Can you work these out from the model? Positions are in its coordinate system, mm. A direction names the side the tool comes from. Coordinates: 2 decimals unless noted, no trailing zeros. Loops run counter-clockwise (first coordinate to the right, second up) from the corner with the lowest first, then second, coordinate; pieces in that order, holes last.
```python
from build123d import *

# Parameters (mm, degrees)
SKETCH_1_W          = 60
SKETCH_1_H          = 65
EXTRUDE_1_DEPTH     = 6
SKETCH_2_W          = 60
SKETCH_2_H          = 6
EXTRUDE_2_DEPTH     = 19
CUT_EXTRUDE_2_REACH = 93.924
SKETCH_4_R          = 3
CUT_EXTRUDE_3_REACH = 93.924
SKETCH_3_R          = 27
SKETCH_3_R_2        = 2


with BuildPart() as part:
    # 草圖1 → 填料-伸長1 (new body)
    with BuildSketch(Plane.XY):
        with Locations((30, 32.5)):
            Rectangle(SKETCH_1_W, SKETCH_1_H)
    extrude(amount=EXTRUDE_1_DEPTH)

    # 草圖2 → 填料-伸長2 (add)
    with BuildSketch(Plane.XY.offset(6)):
        with Locations((30, 3)):
            Rectangle(SKETCH_2_W, SKETCH_2_H)
    extrude(amount=EXTRUDE_2_DEPTH)

    # 草圖4 → 除料-伸長2 (cut, up to next)
    with BuildSketch(Plane(origin=(0, 0, 0), x_dir=(-1, 0, 0), z_dir=(0, -1, 0)), mode=Mode.PRIVATE) as cut_extrude_2_sk1:
        with Locations(Location((-13, -12.5, 0), (0, 0, 90))):
            Circle(SKETCH_4_R)
    cut_extrude_2_tool1 = extrude(cut_extrude_2_sk1.sketch, amount=-CUT_EXTRUDE_2_REACH, mode=Mode.PRIVATE) & part.part
    # 草圖4 → 除料-伸長2 (cut, up to next)
    with BuildSketch(Plane(origin=(0, 0, 0), x_dir=(-1, 0, 0), z_dir=(0, -1, 0)), mode=Mode.PRIVATE) as cut_extrude_2_sk2:
        with Locations(Location((-47, -12.5, 0), (0, 0, 90))):
            Circle(SKETCH_4_R)
    cut_extrude_2_tool2 = extrude(cut_extrude_2_sk2.sketch, amount=-CUT_EXTRUDE_2_REACH, mode=Mode.PRIVATE) & part.part
    add(cut_extrude_2_tool1.solids().sort_by_distance((13, 0, 12.5))[0], mode=Mode.SUBTRACT)
    add(cut_extrude_2_tool2.solids().sort_by_distance((47, 0, 12.5))[0], mode=Mode.SUBTRACT)

    # 草圖3 → 除料-伸長3 (cut, up to next)
    with BuildSketch(Plane(origin=(0, 0, 0), x_dir=(-1, 0, 0), z_dir=(0, 0, -1)), mode=Mode.PRIVATE) as cut_extrude_3_sk1:
        with Locations((-30, 35)):
            Circle(SKETCH_3_R)
    cut_extrude_3_tool1 = extrude(cut_extrude_3_sk1.sketch, amount=-CUT_EXTRUDE_3_REACH, mode=Mode.PRIVATE) & part.part
    # 草圖3 → 除料-伸長3 (cut, up to next)
    with BuildSketch(Plane(origin=(0, 0, 0), x_dir=(-1, 0, 0), z_dir=(0, 0, -1)), mode=Mode.PRIVATE) as cut_extrude_3_sk2:
        with Locations((-54.748737342, 59.748737342)):
            Circle(SKETCH_3_R_2)
    cut_extrude_3_tool2 = extrude(cut_extrude_3_sk2.sketch, amount=-CUT_EXTRUDE_3_REACH, mode=Mode.PRIVATE) & part.part
    # 草圖3 → 除料-伸長3 (cut, up to next)
    with BuildSketch(Plane(origin=(0, 0, 0), x_dir=(-1, 0, 0), z_dir=(0, 0, -1)), mode=Mode.PRIVATE) as cut_extrude_3_sk3:
        with Locations((-5.251262658, 59.748737342)):
            Circle(SKETCH_3_R_2)
    cut_extrude_3_tool3 = extrude(cut_extrude_3_sk3.sketch, amount=-CUT_EXTRUDE_3_REACH, mode=Mode.PRIVATE) & part.part
    # 草圖3 → 除料-伸長3 (cut, up to next)
    with BuildSketch(Plane(origin=(0, 0, 0), x_dir=(-1, 0, 0), z_dir=(0, 0, -1)), mode=Mode.PRIVATE) as cut_extrude_3_sk4:
        with Locations((-54.748737342, 10.251262658)):
            Circle(SKETCH_3_R_2)
    cut_extrude_3_tool4 = extrude(cut_extrude_3_sk4.sketch, amount=-CUT_EXTRUDE_3_REACH, mode=Mode.PRIVATE) & part.part
    # 草圖3 → 除料-伸長3 (cut, up to next)
    with BuildSketch(Plane(origin=(0, 0, 0), x_dir=(-1, 0, 0), z_dir=(0, 0, -1)), mode=Mode.PRIVATE) as cut_extrude_3_sk5:
        with Locations((-5.251262658, 10.251262658)):
            Circle(SKETCH_3_R_2)
    cut_extrude_3_tool5 = extrude(cut_extrude_3_sk5.sketch, amount=-CUT_EXTRUDE_3_REACH, mode=Mode.PRIVATE) & part.part
    add(cut_extrude_3_tool1.solids().sort_by_distance((30, 35, 0))[0], mode=Mode.SUBTRACT)
    add(cut_extrude_3_tool2.solids().sort_by_distance((54.748737, 59.748737, 0))[0], mode=Mode.SUBTRACT)
    add(cut_extrude_3_tool3.solids().sort_by_distance((5.251263, 59.748737, 0))[0], mode=Mode.SUBTRACT)
    add(cut_extrude_3_tool4.solids().sort_by_distance((54.748737, 10.251263, 0))[0], mode=Mode.SUBTRACT)
    add(cut_extrude_3_tool5.solids().sort_by_distance((5.251263, 10.251263, 0))[0], mode=Mode.SUBTRACT)


solid = part.part
```
(1) I want a section at D-D on z = 2.25. Write out the boundary of the cut face in (x, y), then the cut area to 3 significant figures.
Check values:
outline: (0, 0) - (60, 0) - (60, 65) - (0, 65) - close; hole circle Ø54 at (30, 35); hole circle Ø4 at (5.25, 10.25); hole circle Ø4 at (5.25, 59.75); hole circle Ø4 at (54.75, 10.25); hole circle Ø4 at (54.75, 59.75)
area: 1,560 mm2
(2) I'm going to push flat-ended pins straight in: pin 1 (6 mm diameter, centred on x = 40.5, z = 16.5, fed in from +Y); pin 2 (5 mm diameter, centred on x = 13, z = 12.5, fed in from -Y). Where does each tip first touch, or does it pass through?
Check values:
pin 1: stops at y = 6
pin 2: passes through
(3) If I drill on probe 1 along X at (y, z) = (1.35, 12.5); probe 2 along X at (y, z) = (10, 5); probe 3 along Y at (x, z) = (15, 18), over which ranges is the centre line in solid material (lowest first)?
Check values:
probe 1: x = 0 to 10, 16 to 44, 50 to 60
probe 2: x = 0 to 3.27, 7.24 to 19.8, 40.2 to 52.76, 56.73 to 60
probe 3: y = 0 to 6
(4) I want a section at A-A on y = 35. Write out the boundary of the cut face in (x, z), then the cut area to 3 significant figures.
Check values:
outline: (0, 0) - (3, 0) - (3, 6) - (0, 6) - close; (57, 0) - (60, 0) - (60, 6) - (57, 6) - close
area: 36.0 mm2
(5) Which directions (+Z, -Z, +X, -X, +Y, -Y) give clear straight access to the entire face, cutting with the end or side of a thin tool? Please do faces 5 (the flat face through (30, 0, 12)), 6 (the flat face through (23, 62, 6)).
Check values:
face 5: +Z, -Z, +X, -X, -Y
face 6: +Z, +X, -X, +Y
(6) I want a section at C-C on x = 41. Write out the boundary of the cut face in (y, z).
Check values:
outline: (0, 0) - (10.34, 0) - (10.34, 6) - (6, 6) - (6, 25) - (0, 25) - close; (59.66, 0) - (65, 0) - (65, 6) - (59.66, 6) - close
(7) If we mould it in two halves opening along Z, with no side actions, what happens to faces 1 (the flat face through (60, 25, 3)), 2 (the flat face through (30, 3, 25)), 3 (the cylindrical face through (49.974, 2.958, 12.891)), 4 (the cylindrical face through (11.2, 3, 14.9))? For each: released by +Z, released by -Z, zero draft, split by the parting line, or undercut.
Check values:
face 1: zero draft
face 2: released by +Z
face 3: undercut
face 4: undercut
(8) I want a section at B-B on z = 12.5. Write out the boundary of the cut face in (x, y).
Check values:
outline: (0, 0) - (10, 0) - (10, 6) - (0, 6) - close; (16, 0) - (44, 0) - (44, 6) - (16, 6) - close; (50, 0) - (60, 0) - (60, 6) - (50, 6) - close
